from build123d import *

# Parameters (mm, degrees)
CROQUIS1_W              = 80
CROQUIS1_H              = 200
SALIENTE_EXTRUIR1_DEPTH = 5
CROQUIS2_W              = 80
CROQUIS2_H              = 8
SALIENTE_EXTRUIR2_DEPTH = 130
CROQUIS3_R              = 7
CORTAR_EXTRUIR1_DEPTH   = 199.557296517
SALIENTE_EXTRUIR3_DEPTH = 200


with BuildPart() as part:
    # Croquis1 → Saliente-Extruir1 (new body)
    with BuildSketch(Plane(origin=(0, 0, 0), x_dir=(1, 0, 0), z_dir=(0, 1, 0))):
        Rectangle(CROQUIS1_W, CROQUIS1_H)
    saliente_extruir1 = extrude(amount=SALIENTE_EXTRUIR1_DEPTH)

    # Croquis2 → Saliente-Extruir2 (add)
    with BuildSketch(Plane(origin=(0, 5, 0), x_dir=(1, 0, 0), z_dir=(0, 1, 0))):
        with Locations((0, -36)):
            Rectangle(CROQUIS2_W, CROQUIS2_H)
        with Locations((0, 36)):
            Rectangle(CROQUIS2_W, CROQUIS2_H)
    saliente_extruir2 = extrude(amount=SALIENTE_EXTRUIR2_DEPTH)

    # Croquis3 → Cortar-Extruir1 (cut, through all)
    with BuildSketch(Plane.XY.offset(40)):
        with Locations((-9.539199318, 75)):
            Circle(CROQUIS3_R)
    cortar_extruir1 = extrude(amount=-CORTAR_EXTRUIR1_DEPTH, mode=Mode.SUBTRACT)

    # Simetría1: Saliente-Extruir1, Saliente-Extruir2, Cortar-Extruir1 across plane
    add(saliente_extruir1.mirror(Plane(origin=(40, 5, 100), x_dir=(0, 0, 1), z_dir=(-1, 0, 0))))
    add(saliente_extruir2.mirror(Plane(origin=(40, 5, 100), x_dir=(0, 0, 1), z_dir=(-1, 0, 0))))
    add(cortar_extruir1.mirror(Plane(origin=(40, 5, 100), x_dir=(0, 0, 1), z_dir=(-1, 0, 0))), mode=Mode.SUBTRACT)

    # Croquis4 → Saliente-Extruir3 (add)
    with BuildSketch(Plane(origin=(0, 0, -100), x_dir=(-1, 0, 0), z_dir=(0, 0, -1))):
        with BuildLine():
            Line((-6.271231435, -124), (-6.271231435, -7.977831946))
            ThreePointArc((-6.271231435, -7.977831946), (-5.392551778, -5.856511602), (-3.271231435, -4.977831946))
            Line((-3.271231435, -4.977831946), (40.000969046, -4.977831946))
            Line((40.000969046, -4.977831946), (40.000969046, 0))
            Line((40.000969046, 0), (40, 0))
            Line((40, 0), (-7.271231435, 0))
            ThreePointArc((-7.271231435, 0), (-9.392551778, -0.878679656), (-10.271231435, -3))
            Line((-10.271231435, -3), (-10.271231435, -4.977831946))
            Line((-10.271231435, -4.977831946), (-10.271231435, -120))
            Line((-10.271231435, -120), (-70.845112341, -120))
            Line((-70.845112341, -120), (-70.845112341, -4.977831946))
            Line((-70.845112341, -4.977831946), (-70.845112341, -3))
            ThreePointArc((-70.845112341, -3), (-71.723791998, -0.878679656), (-73.845112341, 0))
            Line((-73.845112341, 0), (-119.056976736, 0))
            Line((-119.056976736, 0), (-119.056976736, -4.977831946))
            Line((-119.056976736, -4.977831946), (-77.845112341, -4.977831946))
            ThreePointArc((-77.845112341, -4.977831946), (-75.723791998, -5.856511602), (-74.845112341, -7.977831946))
            Line((-74.845112341, -7.977831946), (-74.845112341, -124))
            Line((-74.845112341, -124), (-6.271231435, -124))
        make_face()
    extrude(amount=-SALIENTE_EXTRUIR3_DEPTH)


solid = part.part
Here's how the part is built. I have some questions about the finished solid (model axes, mm). A direction names the side the tool comes from. Give positions to 0.01 mm unless a question says otherwise; leave off trailing zeros. Loops run counter-clockwise (first coordinate to the right, second up) from the corner with the lowest first, then second, coordinate; pieces in that order, holes last. Notation, with made-up numbers: (2.25, 14) -> (36.25, 14) arc R27 ccw to (36.25, 32) -> close; hole circle Ø4 at (88.5, 42.5). An arc over 180 degrees is marked (long way). Answer as a JSON object with one key per item and string values. Group by question number.
Item 1: I need wall thicknesses on L1, parallel to Z at x = 62.5, y = 66.5; L2, parallel to X at y = -24.5, z = 84.5; L3, parallel to Y at x = 63, z = -27.5. Which ranges of each line are inside material? Lowest first, please.
Item 2: On a 3-axis mill with a long thin cutter (end or side, diameter ignored), from which of +Z, -Z, +X, -X, +Y, -Y can I reach the whole of each face in a straight line? I mean faces 5 (the flat face through (41, 69, 32)), 6 (the flat face through (41, 5, -70)), 7 (the flat face through (6.271, -67, -1)), 8 (the flat face through (10.271, -61, -1)), 9 (the flat face through (99, -4.978, -1)). Say none if no direction works.
Item 3: Will these pins go through, and if not, where does the flat tip stop? pin 1 (22.5 mm diameter, centred on x = -9.54, y = 75, fed in from +Z); pin 2 (2.5 mm diameter, centred on y = -2, z = -19.5, fed in from +X); pin 3 (4 mm diameter, centred on x = -2.5, z = 52.5, fed in from +Y).
Item 4: Thinking about a two-plate mould opening in Z: for faces 1 (the flat face through (41, 69, -32)), 2 (the flat face through (41, 69, -40)), 3 (the flat face through (41, 5, 0)), 4 (the flat face through (41, 69, 40)), which applies, pulls with the +Z half, pulls with the -Z half, needs draft (parallel to the pull), parting line crosses it, or undercut?
Item 5: Imagine slicing it at A-A on y = 75. Write out the boundary of the cut face in (x, z).
Item 6: Imagine slicing it at B-B on z = -35. Give the number of separate pieces and of enclosed holes in the cut face, then the cut area to 3 significant figures.
Item 7: Imagine slicing it at C-C on y = -24. Write out the boundary of the cut face in (x, z), then the cut area to 3 significant figures.
Answer list:
{
 "1": {"L1": "z = -40 to -32, 32 to 40", "L2": "x = 6.27 to 10.27, 70.85 to 74.85", "L3": "y = -124 to -120, 0 to 5"},
 "2": {"face 5": "+X, -X, +Y", "face 6": "-Z, +X, -X, +Y", "face 7": "+Z, -Z, -X, -Y", "face 8": "+Z, -Z", "face 9": "+Z, -Z, +X, -Y"},
 "3": {"pin 1": "stops at z = 40", "pin 2": "stops at x = 119.06", "pin 3": "stops at y = 5"},
 "4": {"face 1": "undercut", "face 2": "pulls with the -Z half", "face 3": "undercut", "face 4": "pulls with the +Z half"},
 "5": {"outline": "(-40, -40) -> (-16.54, -40) -> (-16.54, -32) -> (-40, -32) -> close; (-40, 32) -> (-16.54, 32) -> (-16.54, 40) -> (-40, 40) -> close; (-2.54, -40) -> (82.54, -40) -> (82.54, -32) -> (-2.54, -32) -> close; (-2.54, 32) -> (82.54, 32) -> (82.54, 40) -> (-2.54, 40) -> close; (96.54, -40) -> (120, -40) -> (120, -32) -> (96.54, -32) -> close; (96.54, 32) -> (120, 32) -> (120, 40) -> (96.54, 40) -> close"},
 "6": {"separate pieces": "1", "enclosed holes": "3", "area": "23,000 mm2"},
 "7": {"outline": "(6.27, -100) -> (10.27, -100) -> (10.27, 100) -> (6.27, 100) -> close; (70.85, -100) -> (74.85, -100) -> (74.85, 100) -> (70.85, 100) -> close", "area": "1,600 mm2"}
}
